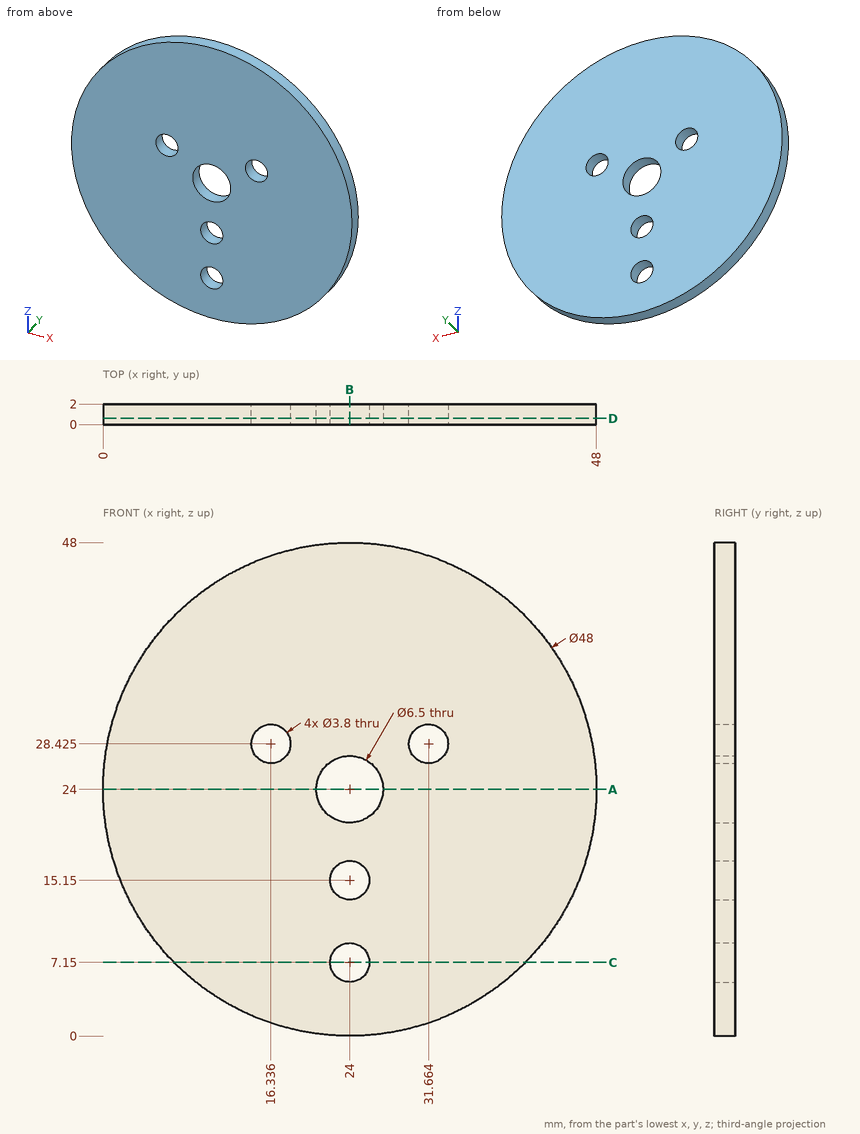
Source: three-view drawing plus pictorial views. Frame: mm from the lowest corner of the part. Round coordinates to 2 decimals unless told otherwise and drop trailing zeros. Loops run counter-clockwise (first coordinate to the right, second up) from the corner with the lowest first, then second, coordinate; pieces in that order, holes last.
1. Section query D-D on y = 0.6. Give the number of separate pieces and of enclosed holes in the cut face, and give its area (3 significant figures).
2. Contact query for a flat-ended pin moving along its axis: pin 1 (3 mm diameter, centred on x = 31.66, z = 28.42, fed in from -Y). Output: stop coordinate, or through.
3. Section query C-C on z = 7.15. Output: boundary loops of the cut face in (x, y).
4. Section query A-A on z = 24. Output: boundary loops of the cut face in (x, y).
5. Ray query, L1, parallel to Z at x = 24, y = 1.1; L2, parallel to X at y = 0.95, z = 24; L3, parallel to Z at x = 25, y = 1.5 (1 decimal). Return the intervals inside material, ascending.
6. Section query B-B on x = 24. Output: boundary loops of the cut face in (y, z).
Answers below:
1. separate pieces: 1
1. enclosed holes: 5
1. area: 1,730 mm2
2. pin 1: passes through
3. outline: (6.91, 0) - (22.1, 0) - (22.1, 2) - (6.91, 2) - close; (25.9, 0) - (41.09, 0) - (41.09, 2) - (25.9, 2) - close
4. outline: (0, 0) - (20.75, 0) - (20.75, 2) - (0, 2) - close; (27.25, 0) - (48, 0) - (48, 2) - (27.25, 2) - close
5. L1: z = 0 to 5.25, 9.05 to 13.25, 17.05 to 20.75, 27.25 to 48
5. L2: x = 0 to 20.75, 27.25 to 48
5. L3: z = 0 to 5.5, 8.8 to 13.5, 16.8 to 20.9, 27.1 to 48
6. outline: (0, 0) - (2, 0) - (2, 5.25) - (0, 5.25) - close; (0, 9.05) - (2, 9.05) - (2, 13.25) - (0, 13.25) - close; (0, 17.05) - (2, 17.05) - (2, 20.75) - (0, 20.75) - close; (0, 27.25) - (2, 27.25) - (2, 48) - (0, 48) - close
